Check sheet for the drawn part. Datum: minimum x, y, z corner. Units: mm. A direction names the side the tool comes from. Coordinates: 2 decimals unless noted, no trailing zeros. Write each loop counter-clockwise with the first axis right and the second up, starting at its lowest first coordinate (ties: lowest second). Pieces come first, ordered by that corner, then holes. Notation, with made-up numbers: (88.5, -3.5) - (147.5, -3.5) arc R24 cw to (147.5, 29.5) - close; hole circle Ø3 at (57, -6). An arc over 180 degrees is marked (long way). Use one line per item in the form item = value. Start each with the question number.
1. Go/stop test with flat-tipped pins: pin 1 Ø1.1 at (x, y) = (65, 14.5) entering from +Z; pin 2 Ø3 at (x, z) = (40.5, 20) entering from +Y; pin 3 Ø5 at (x, z) = (42, 56) entering from +Y; pin 4 Ø3 at (x, z) = (2.5, 2.5) entering from -Y. Record where each tip stops, or that it passes through.
2. Cross-section at C-C on z = 31.5. Record the boundary of the cut face in (x, y).
3. Draft check along Z on the marked faces 4, 5 and 6. Enter one of: +Z half, -Z half, draft (parallel to the pull), parting line (faces both ways), or undercut.
4. Tool access check on the marked faces 1, 2 and 3. Record the directions out of +Z, -Z, +X, -X, +Y, -Y that give a thin tool (end or side, any length) a straight path to the whole face; none if there is none.
5. Cross-section at B-B on z = 57.5. Record the boundary of the cut face in (x, y), then the cut area to 3 significant figures.
6. Scan lines: line 1 along Z through (x, y) = (95.5, 0.8); line 2 along X through (y, z) = (0.75, 2.5); line 3 along Z through (x, y) = (30.5, 14.25). Record each from-to range of solid material in increasing order.
7. Cross-section at D-D on x = 26.5. Record the boundary of the cut face in (y, z), then the cut area to 3 significant figures.
8. Cross-section at A-A on x = 95.5. Record the boundary of the cut face in (y, z).
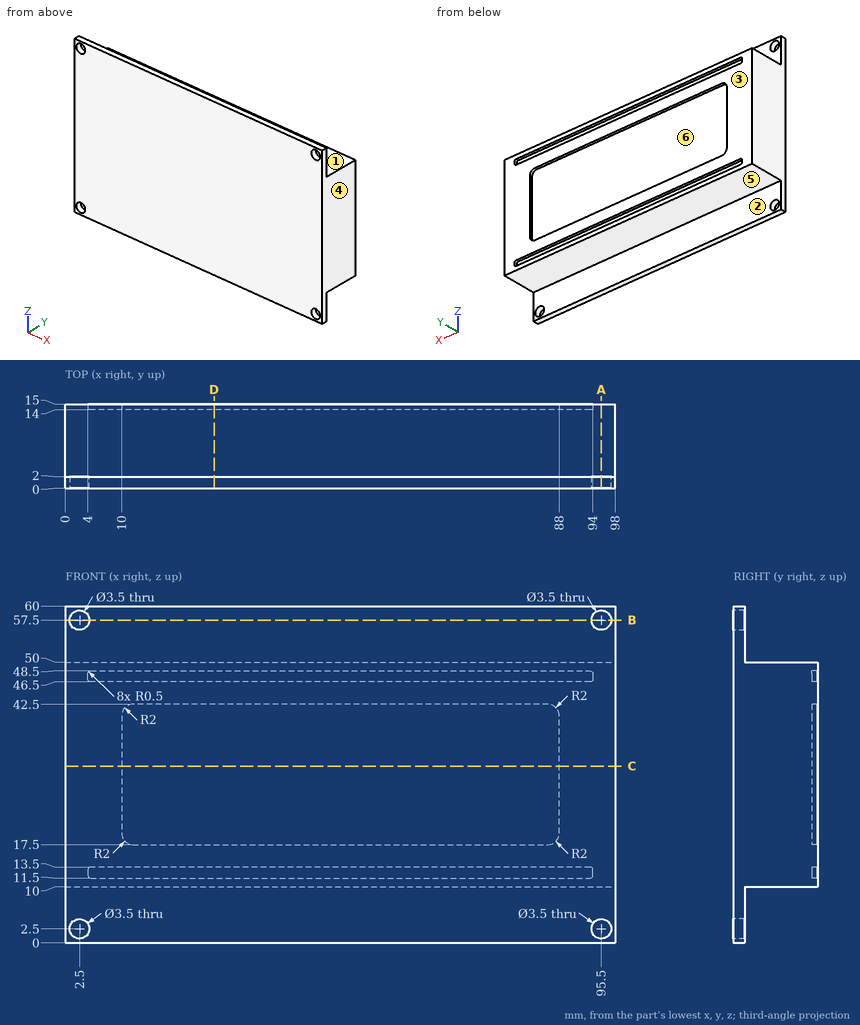
Final values:
q1.pin_1 = 50
q1.pin_2 = 14
q1.pin_3 = 2
q1.pin_4 = through
q2.outline = (0, 0) - (98, 0) - (98, 15) - (88, 15) - (88, 14) - (10, 14) - (10, 15) - (0, 15) - close
q3.face_4 = draft
q3.face_5 = -Z half
q3.face_6 = undercut
q4.face_1 = +Z, +X, -X, +Y
q4.face_2 = -Z, +X, -X, +Y
q4.face_3 = +Z, -Z, +X, -X, +Y
q5.outline = (0, 0) - (0.75, 0) - (0.75, 2) - (0, 2) - close; (4.25, 0) - (93.75, 0) - (93.75, 2) - (4.25, 2) - close; (97.25, 0) - (98, 0) - (98, 2) - (97.25, 2) - close
q5.area = 182 mm²
q6.line_1 = 0 to 0.75, 4.25 to 55.75, 59.25 to 60
q6.line_2 = 0 to 0.75, 4.25 to 93.75, 97.25 to 98
q6.line_3 = 10 to 11.5, 13.5 to 17.5, 42.5 to 46.5, 48.5 to 50
q7.outline = (0, 0) - (2, 0) - (2, 10) - (15, 10) - (15, 11.5) - (14, 11.5) - (14, 13.5) - (15, 13.5) - (15, 17.5) - (14, 17.5) - (14, 42.5) - (15, 42.5) - (15, 46.5) - (14, 46.5) - (14, 48.5) - (15, 48.5) - (15, 50) - (2, 50) - (2, 60) - (0, 60) - close
q7.area = 611 mm²
q8.outline = (0, 0) - (2, 0) - (2, 0.75) - (0, 0.75) - close; (0, 4.25) - (2, 4.25) - (2, 10) - (15, 10) - (15, 50) - (2, 50) - (2, 55.75) - (0, 55.75) - close; (0, 59.25) - (2, 59.25) - (2, 60) - (0, 60) - close
